Part print with two shaded views. Sizes in mm from the minimum x, y, z corner. Coordinates: 2 decimals unless noted, no trailing zeros. Order: outer loops, then holes, each group sorted by start corner. A loop starts at its lowest first (then second) coordinate and runs counter-clockwise, first axis right, second up. Notation, with made-up numbers: (3, 8) - (10, 8) arc R5 ccw to (10, 16) - close; hole circle Ø5 at (-23, 30.5). An arc over 180 degrees is marked (long way). One line per item, written item: value.
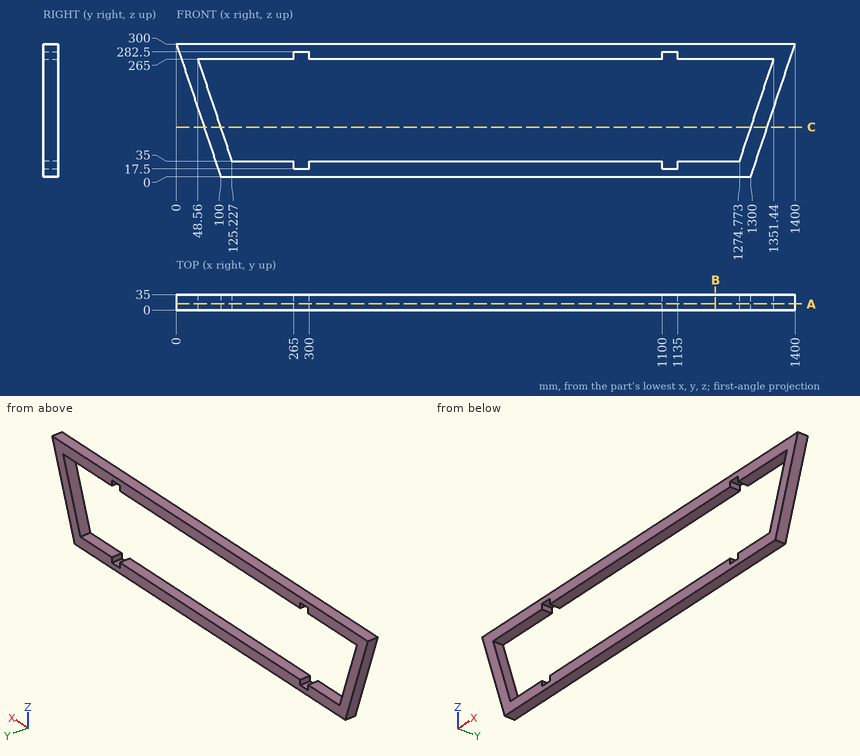
1. Band-saw the part on A-A, the plane y = 14. Give the cut face in (x, z).
Values found:
outline: (0, 300) - (100, 0) - (1300, 0) - (1400, 300) - close; hole (48.56, 265) - (125.23, 35) - (265, 35) - (265, 17.5) - (300, 17.5) - (300, 35) - (1100, 35) - (1100, 17.5) - (1135, 17.5) - (1135, 35) - (1274.77, 35) - (1351.44, 265) - (1135, 265) - (1135, 282.5) - (1100, 282.5) - (1100, 265) - (300, 265) - (300, 282.5) - (265, 282.5) - (265, 265) - close
2. Probe line 1 along Z through (x, y) = (845, 18.5); line 2 along X through (y, z) = (30.5, 106.5); line 3 along X through (y, z) = (2, 84). List the from-to ranges inside material, lowest first.
Values found:
line 1: z = 0 to 35, 265 to 300
line 2: x = 64.5 to 101.39, 1298.61 to 1335.5
line 3: x = 72 to 108.89, 1291.11 to 1328
3. Band-saw the part on C-C, the plane z = 112. Give the cut face in (x, y).
Values found:
outline: (62.67, 0) - (99.56, 0) - (99.56, 35) - (62.67, 35) - close; (1300.44, 0) - (1337.33, 0) - (1337.33, 35) - (1300.44, 35) - close
4. Band-saw the part on B-B, the plane x = 1220. Give the cut face in (y, z), and give its area (3 significant figures).
Values found:
outline: (0, 0) - (35, 0) - (35, 35) - (0, 35) - close; (0, 265) - (35, 265) - (35, 300) - (0, 300) - close
area: 2,450 mm2
5. Flat gauge pins, fed straight in: P1, Ø12, axis at y = 10, z = 201, coming from the -X side; P2, Ø9, axis at y = 18.5, z = 22.5, coming from the +X side; P3, Ø6, axis at y = 10.5, z = 180.5, coming from the +X side. Where does each tip first touch, or does it go through?
Values found:
P1: stops at x = 31
P2: stops at x = 1309
P3: stops at x = 1361.17
